Here's how the part is built. I have some questions about the finished solid (model axes, mm). A direction names the side the tool comes from. Round coordinates to 2 decimals unless told otherwise and drop trailing zeros. Order: outer loops, then holes, each group sorted by start corner. A loop starts at its lowest first (then second) coordinate and runs counter-clockwise, first axis right, second up. Notation, with made-up numbers: (-34, 35.5) - (-9, 35.5) arc R17 ccw to (-9, 52.5) - close; hole circle Ø5 at (25.25, 37). An arc over 180 degrees is marked (long way). One line per item, written item: value.
from build123d import *

# Parameters (mm, degrees)
F1_DEPTH  = 12.7
F2_R      = 39.37
F3_DEPTH  = 12.7
F5_DEPTH  = 6.35
F6_R      = 63.5
F6_R_2    = 39.37
F7_DEPTH  = 6.35
F9_DEPTH  = 3.175
F10_R     = 39.37
F11_DEPTH = 3.175
F12_R     = 19.05
F12_R_2   = 12.7
F13_DEPTH = 6.35


with BuildPart() as f1:
    # F0 (on Top) → F1 (new body)
    with BuildSketch(Plane.XY):
        with BuildLine():
            Line((-42.8625, 122.2375), (-42.8625, 105.958936))
            ThreePointArc((-42.8625, 105.958936), (-80.822305, 80.822305), (-105.958936, 42.8625))
            ThreePointArc((-105.958936, 42.8625), (-114.3, 0), (-105.958936, -42.8625))
            ThreePointArc((-105.958936, -42.8625), (-80.822305, -80.822305), (-42.8625, -105.958936))
            ThreePointArc((-42.8625, -105.958936), (0, -114.3), (42.8625, -105.958936))
            ThreePointArc((42.8625, -105.958936), (80.822305, -80.822305), (105.958936, -42.8625))
            Line((105.958936, -42.8625), (122.2375, -42.8625))
            Line((122.2375, -42.8625), (122.2375, 42.8625))
            Line((122.2375, 42.8625), (105.958936, 42.8625))
            ThreePointArc((105.958936, 42.8625), (80.822305, 80.822305), (42.8625, 105.958936))
            Line((42.8625, 105.958936), (42.8625, 122.2375))
            Line((42.8625, 122.2375), (-42.8625, 122.2375))
        make_face()
        with BuildLine():
            ThreePointArc((-105.958936, -42.8625), (-114.3, 0), (-105.958936, 42.8625))
            Line((-105.958936, 42.8625), (-122.2375, 42.8625))
            Line((-122.2375, 42.8625), (-122.2375, -42.8625))
            Line((-122.2375, -42.8625), (-105.958936, -42.8625))
        make_face()
        with BuildLine():
            ThreePointArc((42.8625, -105.958936), (0, -114.3), (-42.8625, -105.958936))
            Line((-42.8625, -105.958936), (-42.8625, -122.2375))
            Line((-42.8625, -122.2375), (42.8625, -122.2375))
            Line((42.8625, -122.2375), (42.8625, -105.958936))
        make_face()
    extrude(amount=F1_DEPTH)

    # F2 (on face) → F3 (cut, through all)
    with BuildSketch(Plane.XY.offset(12.7)):
        Circle(F2_R)
    extrude(amount=-F3_DEPTH, mode=Mode.SUBTRACT)

    # F4 (on face) → F5 (cut)
    with BuildSketch(Plane.XY.offset(12.7)):
        Polygon((31.75, 114.3), (-31.75, 114.3), (-31.75, 31.75), (-114.3, 31.75), (-114.3, -31.75), (-31.75, -31.75), (-31.75, -42.8625), (-31.75, -114.3), (31.75, -114.3), (31.75, -42.8625), (31.75, -31.75), (42.8625, -31.75), (114.3, -31.75), (114.3, 31.75), (31.75, 31.75), align=None)
        with BuildLine():
            Line((-42.8625, -42.8625), (-99.075772, -42.8625))
            ThreePointArc((-99.075772, -42.8625), (-76.332177, -76.332177), (-42.8625, -99.075772))
            Line((-42.8625, -99.075772), (-42.8625, -42.8625))
        make_face()
        with BuildLine():
            Line((42.8625, 42.8625), (99.075772, 42.8625))
            ThreePointArc((99.075772, 42.8625), (76.332177, 76.332177), (42.8625, 99.075772))
            Line((42.8625, 99.075772), (42.8625, 42.8625))
        make_face()
        with BuildLine():
            Line((-42.8625, 42.8625), (-42.8625, 99.075772))
            ThreePointArc((-42.8625, 99.075772), (-76.332177, 76.332177), (-99.075772, 42.8625))
            Line((-99.075772, 42.8625), (-42.8625, 42.8625))
        make_face()
        with BuildLine():
            Line((42.8625, -42.8625), (42.8625, -99.075772))
            ThreePointArc((42.8625, -99.075772), (76.332177, -76.332177), (99.075772, -42.8625))
            Line((99.075772, -42.8625), (42.8625, -42.8625))
        make_face()
    extrude(amount=-F5_DEPTH, mode=Mode.SUBTRACT)

    # F6 (on face) → F7 (join)
    with BuildSketch(Plane.XY.offset(6.35)):
        Circle(F6_R)
        Circle(F6_R_2, mode=Mode.SUBTRACT)
    extrude(amount=F7_DEPTH)

    # F8 (on face) → F9 (join)
    with BuildSketch(Plane.XY.offset(12.7)):
        Polygon((3.656339, 46.667791), (0, 61.695147), (-3.689128, 46.665211), (-9.651247, 60.935578), (-10.943756, 45.513578), (-19.064849, 58.675572), (-17.928912, 43.24125), (-28.009011, 54.970779), (-24.472599, 39.904178), (-36.263498, 49.912423), (-30.41369, 35.584534), (-43.625057, 43.625057), (-35.605894, 30.38868), (-49.912423, 36.263498), (-39.921364, 24.444555), (-54.970779, 28.009011), (-43.253836, 17.898525), (-58.675572, 19.064849), (-45.521256, 10.911774), (-60.935578, 9.651247), (-46.667791, 3.656339), (-61.695147, 0), (-46.665211, -3.689128), (-60.935578, -9.651247), (-45.513578, -10.943756), (-58.675572, -19.064849), (-43.24125, -17.928912), (-54.970779, -28.009011), (-39.904178, -24.472599), (-49.912423, -36.263498), (-35.584534, -30.41369), (-43.625057, -43.625057), (-30.38868, -35.605894), (-36.263498, -49.912423), (-24.444555, -39.921364), (-28.009011, -54.970779), (-17.898525, -43.253836), (-19.064849, -58.675572), (-10.911774, -45.521256), (-9.651247, -60.935578), (-3.656339, -46.667791), (0, -61.695147), (3.689128, -46.665211), (9.651247, -60.935578), (10.943756, -45.513578), (19.064849, -58.675572), (17.928912, -43.24125), (28.009011, -54.970779), (24.472599, -39.904178), (36.263498, -49.912423), (30.41369, -35.584534), (43.625057, -43.625057), (35.605894, -30.38868), (49.912423, -36.263498), (39.921364, -24.444555), (54.970779, -28.009011), (43.253836, -17.898525), (58.675572, -19.064849), (45.521256, -10.911774), (60.935578, -9.651247), (46.667791, -3.656339), (61.695147, 0), (46.665211, 3.689128), (60.935578, 9.651247), (45.513578, 10.943756), (58.675572, 19.064849), (43.24125, 17.928912), (54.970779, 28.009011), (39.904178, 24.472599), (49.912423, 36.263498), (35.584534, 30.41369), (43.625057, 43.625057), (30.38868, 35.605894), (36.263498, 49.912423), (24.444555, 39.921364), (28.009011, 54.970779), (17.898525, 43.253836), (19.064849, 58.675572), (10.911774, 45.521256), (9.651247, 60.935578), align=None)
    extrude(amount=F9_DEPTH)

    # F10 (on face) → F11 (cut, through all)
    with BuildSketch(Plane.XY.offset(15.875)):
        Circle(F10_R)
    extrude(amount=-F11_DEPTH, mode=Mode.SUBTRACT)

    # F12 (on face) → F13 (join)
    with BuildSketch(Plane.XY.offset(12.7)):
        with Locations((0, 87.997574)):
            Circle(F12_R)
        with Locations((60.616729, 60.616729)):
            Circle(F12_R_2)
        with Locations((88.9, 0)):
            Circle(F12_R)
        with Locations((60.616729, -60.616729)):
            Circle(F12_R_2)
        with Locations((0, -88.9)):
            Circle(F12_R)
        with Locations((-59.978617, -61.237198)):
            Circle(F12_R_2)
        with Locations((-88.9, 0)):
            Circle(F12_R)
        with Locations((-60.616729, 60.616729)):
            Circle(F12_R_2)
    extrude(amount=-F13_DEPTH)


solid = f1.part
Q1. If we section it at B-B, the plane x = -88.9: Please give me the cut outline in (y, z), then the cut area to 3 significant figures.
Results list:
outline: (-71.84, 0) - (71.84, 0) - (71.84, 12.7) - (61.24, 12.7) - (61.24, 6.35) - (42.86, 6.35) - (42.86, 12.7) - (31.75, 12.7) - (31.75, 6.35) - (19.05, 6.35) - (19.05, 12.7) - (-19.05, 12.7) - (-19.05, 6.35) - (-31.75, 6.35) - (-31.75, 12.7) - (-42.86, 12.7) - (-42.86, 6.35) - (-61.24, 6.35) - (-61.24, 12.7) - (-71.84, 12.7) - close
area: 1,430 mm²
Q2. Will these pins go through, and if not, where does the flat tip stop? pin 1 (3 mm diameter, centred on y = 95.5, z = 13.5, fed in from -X); pin 2 (7.5 mm diameter, centred on x = -64.5, y = -55, fed in from +Z); pin 3 (4 mm diameter, centred on x = 111.5, z = 9.5, fed in from -Y).
Results list:
pin 1: x = -64.69
pin 2: z = 12.7
pin 3: y = -42.86
Q3. If we section it at C-C, the plane y = 78.5: Please give me the cut outline in (x, z), then the cut area to 3 significant figures.
Results list:
outline: (-83.08, 0) - (83.08, 0) - (83.08, 12.7) - (74.1, 12.7) - (74.1, 6.35) - (42.86, 6.35) - (42.86, 12.7) - (31.75, 12.7) - (31.75, 6.35) - (16.51, 6.35) - (16.51, 12.7) - (-16.51, 12.7) - (-16.51, 6.35) - (-31.75, 6.35) - (-31.75, 12.7) - (-42.86, 12.7) - (-42.86, 6.35) - (-74.1, 6.35) - (-74.1, 12.7) - (-83.08, 12.7) - close
area: 1,520 mm²
Q4. If I drill on line 1 along Y through (x, z) = (0, 12.5); line 2 along X through (y, z) = (110, 9); line 3 along Y through (x, z) = (0, 4.75), over which ranges is the centre line in solid material (lowest first)?
Results list:
line 1: -122.24 to -114.3, -107.95 to -69.85, -63.5 to -39.37, 39.37 to 63.5, 68.95 to 107.05, 114.3 to 122.24
line 2: -42.86 to -31.75, 31.75 to 42.86
line 3: -122.24 to -39.37, 39.37 to 122.24
Q5. Which directions (+Z, -Z, +X, -X, +Y, -Y) give clear straight access to the entire face, cutting with the end or side of a thin tool? Please do faces 1 (the flat face through (-114, -42.862, 6)), 2 (the flat face through (71, -71, 6.35)), 3 (the flat face through (114, 42.862, 6)).
Results list:
face 1: +Z, -Z, -X, -Y
face 2: +Z
face 3: +Z, -Z, +X, +Y
Q6. If we section it at A-A, the plane z = 3.5: Please give me the cut outline in (x, y).
Results list:
outline: (-122.24, -42.86) - (-105.96, -42.86) arc R114.3 ccw to (-42.86, -105.96) - (-42.86, -122.24) - (42.86, -122.24) - (42.86, -105.96) arc R114.3 ccw to (105.96, -42.86) - (122.24, -42.86) - (122.24, 42.86) - (105.96, 42.86) arc R114.3 ccw to (42.86, 105.96) - (42.86, 122.24) - (-42.86, 122.24) - (-42.86, 105.96) arc R114.3 ccw to (-105.96, 42.86) - (-122.24, 42.86) - close; hole circle Ø78.74 at (0, 0)
